```python
from build123d import *

# Parameters (mm, degrees)
SKETCH_1_W          = 50
SKETCH_1_H          = 40
EXTRUDE_1_DEPTH     = 8
CUT_EXTRUDE_1_DEPTH = 2
SKETCH_3_R          = 3.25
CUT_EXTRUDE_2_DEPTH = 10
SKETCH_4_R          = 1.65
CUT_EXTRUDE_3_DEPTH = 15


with BuildPart() as part:
    # Эскиз1 → Бобышка-Вытянуть1 (new body)
    with BuildSketch(Plane.XY):
        Rectangle(SKETCH_1_W, SKETCH_1_H)
    extrude(amount=EXTRUDE_1_DEPTH)

    # Эскиз2 → Вырез-Вытянуть1 (cut)
    with BuildSketch(Plane.XY.offset(8)):
        with BuildLine():
            Line((-6, 5.05), (6, 5.05))
            ThreePointArc((6, 5.05), (11.05, 0), (6, -5.05))
            Line((6, -5.05), (-6, -5.05))
            ThreePointArc((-6, -5.05), (-11.05, 0), (-6, 5.05))
        make_face()
    extrude(amount=-CUT_EXTRUDE_1_DEPTH, mode=Mode.SUBTRACT)

    # Эскиз3 → Вырез-Вытянуть2 (cut)
    with BuildSketch(Plane.XY.offset(6)):
        Circle(SKETCH_3_R)
    extrude(amount=-CUT_EXTRUDE_2_DEPTH, mode=Mode.SUBTRACT)

    # Эскиз4 → Вырез-Вытянуть3 (cut)
    with BuildSketch(Plane(origin=(25, 0, 0), x_dir=(0, 0, -1), z_dir=(1, 0, 0))):
        with Locations(Location((-4, -10, 0), (0, 0, 90))):
            Circle(SKETCH_4_R)
        with Locations(Location((-4, 10, 0), (0, 0, 90))):
            Circle(SKETCH_4_R)
    extrude(amount=-CUT_EXTRUDE_3_DEPTH, mode=Mode.SUBTRACT)


solid = part.part
```
The listing builds one solid part. Answer for the finished solid, in the listing's coordinates (mm). A direction names the side the tool comes from. Give positions to 0.01 mm unless a question says otherwise; leave off trailing zeros. Order: outer loops, then holes, each group sorted by start corner. A loop starts at its lowest first (then second) coordinate and runs counter-clockwise, first axis right, second up.
Item 1: Which of the six approach directions +Z, -Z, +X, -X, +Y, -Y give full straight-line access (tool end or side, diameter ignored) to faces 1 (the face through (0, 9, 8)), 2 (the face through (0, 5.05, 7)), 3 (the face through (17.605, 11.524, 3.368))?
From the geometry:
face 1: +Z, +X, -X, +Y, -Y
face 2: +Z
face 3: +X
Item 2: The part is cut by section C-C, the plane x = -1. Give the vertices of the cut face in (y, z), and give its area (3 significant figures).
From the geometry:
outline: (-20, 0) - (-3.09, 0) - (-3.09, 6) - (-5.05, 6) - (-5.05, 8) - (-20, 8) - close; (3.09, 0) - (20, 0) - (20, 8) - (5.05, 8) - (5.05, 6) - (3.09, 6) - close
area: 263 mm2
Item 3: The part is cut by section D-D, the plane y = 10. Give the vertices of the cut face in (x, z), and give its area (4 significant figures).
From the geometry:
outline: (-25, 0) - (25, 0) - (25, 2.35) - (10, 2.35) - (10, 5.65) - (25, 5.65) - (25, 8) - (-25, 8) - close
area: 350.5 mm2
Item 4: For a pull along Z with two mould halves and no side action, classify faces 4 (the face through (0, 5, 0)), 5 (the face through (11.05, 0.11, 7.01)), 6 (the face through (17.605, -8.476, 3.368)) as pulls with the +Z half, pulls with the -Z half, needs draft (parallel to the pull), parting line crosses it, or undercut.
From the geometry:
face 4: pulls with the -Z half
face 5: needs draft
face 6: undercut
Item 5: Find the intervals of material crossed by probe 1 along Z at (x, y) = (16, -10); probe 2 along Y at (x, z) = (4.5, 6.75); probe 3 along Y at (x, z) = (0, 4), in increasing order.
From the geometry:
probe 1: z = 0 to 2.35, 5.65 to 8
probe 2: y = -20 to -5.05, 5.05 to 20
probe 3: y = -20 to -3.25, 3.25 to 20
Item 6: The part is cut by section A-A, the plane y = 0. Give the vertices of the cut face in (x, z), and give its area (3 significant figures).
From the geometry:
outline: (-25, 0) - (-3.25, 0) - (-3.25, 6) - (-11.05, 6) - (-11.05, 8) - (-25, 8) - close; (3.25, 0) - (25, 0) - (25, 8) - (11.05, 8) - (11.05, 6) - (3.25, 6) - close
area: 317 mm2
Item 7: The part is cut by section B-B, the plane z = 4. Give the vertices of the cut face in (x, y).
From the geometry:
outline: (-25, -20) - (25, -20) - (25, -11.65) - (10, -11.65) - (10, -8.35) - (25, -8.35) - (25, 8.35) - (10, 8.35) - (10, 11.65) - (25, 11.65) - (25, 20) - (-25, 20) - close; hole circle Ø6.5 at (0, 0)
Item 8: Given pin 1 Ø3 at (x, y) = (-1.5, 2) entering from +Z; pin 2 Ø6 at (x, y) = (0, 0) entering from +Z; pin 3 Ø1 at (y, z) = (10.5, 3.5) entering from +X, each flat-ended and moving along its own axis, determine where each tip first touches the part or whether it passes through.
From the geometry:
pin 1: stops at z = 6
pin 2: passes through
pin 3: stops at x = 10
